Check sheet for the modelled part. Datum: model origin and axes. Units: mm. A direction names the side the tool comes from. Coordinates: 2 decimals unless noted, no trailing zeros. Order: outer loops, then holes, each group sorted by start corner. A loop starts at its lowest first (then second) coordinate and runs counter-clockwise, first axis right, second up.
from build123d import *

# Parameters (mm, degrees)
BOSS_EXTRUDE1_DEPTH     = 2.999994
SKETCH3_R               = 3.375082345
SKETCH3_R_2             = 2.3700486
BOSS_EXTRUDE2_DEPTH     = 3.302
SKETCH4_R               = 2.3700486
SKETCH4_R_2             = 1.524
BOSS_EXTRUDE3_DEPTH     = 2.237994
SKETCH5_R               = 3.556
SKETCH5_R_2             = 1.524049463
BOSS_EXTRUDE4_DEPTH     = 1.016
SKETCH6_R               = 1.524049463
CUT_EXTRUDE2_DEPTH      = 20.69939547
CUT_EXTRUDE3_START      = -4.015994
CUT_EXTRUDE3_OUTLINE_R  = 0.621776252
CUT_EXTRUDE3_DEPTH      = 4.015994
CUT_EXTRUDE4_DEPTH      = 21.047545727
CUT_EXTRUDE4_DEPTH_BACK = 3.302
SKETCH9_R               = 3.375082345
SKETCH10_R              = 2.54
CUT_EXTRUDE5_DEPTH      = 20.091339956


# Read off the part's stored shape, not the designer's step: Cut-Extrude3
with BuildPart() as part:
    # Sketch1 → Boss-Extrude1 (new body)
    with BuildSketch(Plane(origin=(0, 0, 0), x_dir=(1, 0, 0), z_dir=(0, 1, 0))):
        with BuildLine():
            Line((-14.960824333, 6.251943389), (-1.121532733, 7.748689189))
            ThreePointArc((-1.121532733, 7.748689189), (-0.719755533, 7.770352511), (-0.317978333, 7.748689189))
            Line((-0.317978333, 7.748689189), (13.521313267, 6.251943389))
            ThreePointArc((13.521313267, 6.251943389), (15.530246603, 4.014889189), (13.521313267, 1.777834989))
            Line((13.521313267, 1.777834989), (-0.317978333, 0.281089189))
            ThreePointArc((-0.317978333, 0.281089189), (-0.719755533, 0.259425867), (-1.121532733, 0.281089189))
            Line((-1.121532733, 0.281089189), (-14.960824333, 1.777834989))
            ThreePointArc((-14.960824333, 1.777834989), (-16.96975767, 4.014889189), (-14.960824333, 6.251943389))
        make_face()
    extrude(amount=BOSS_EXTRUDE1_DEPTH)

    # Sketch3 → Boss-Extrude2 (add)
    with BuildSketch(Plane(origin=(0, 2.999994, 0), x_dir=(1, 0, 0), z_dir=(0, 1, 0))):
        with Locations(Location((-0.719755307, 4.013536412, 0), (0, 0, 90))):
            Circle(SKETCH3_R)
        with Locations(Location((-0.719755307, 4.013536412, 0), (0, 0, 90))):
            Circle(SKETCH3_R_2, mode=Mode.SUBTRACT)
    extrude(amount=BOSS_EXTRUDE2_DEPTH)

    # Sketch4 → Boss-Extrude3 (add)
    with BuildSketch(Plane.XZ):
        with Locations(Location((-0.719755307, -4.013536412, 0), (0, 0, 270))):
            Circle(SKETCH4_R)
        with Locations((-0.719755307, -4.013536412)):
            Circle(SKETCH4_R_2, mode=Mode.SUBTRACT)
    extrude(amount=-BOSS_EXTRUDE3_DEPTH)

    # Sketch5 → Boss-Extrude4 (add)
    with BuildSketch(Plane.XZ):
        with Locations(Location((-0.7197993, -4.014912249, 0), (0, 0, 270))):
            Circle(SKETCH5_R)
        with Locations(Location((-0.7197993, -4.014912249, 0), (0, 0, 270))):
            Circle(SKETCH5_R_2, mode=Mode.SUBTRACT)
    extrude(amount=BOSS_EXTRUDE4_DEPTH)

    # Sketch6 → Cut-Extrude2 (cut, through all)
    with BuildSketch(Plane.XZ):
        with Locations(Location((-0.7197993, -4.014912249, 0), (0, 0, 270))):
            Circle(SKETCH6_R)
    extrude(amount=-CUT_EXTRUDE2_DEPTH, mode=Mode.SUBTRACT)

    # Cut-Extrude3 outline → Cut-Extrude3 (cut)
    with BuildSketch(Plane(origin=(0, 2.999994, 0), x_dir=(1, 0, 0), z_dir=(0, 1, 0)).offset(CUT_EXTRUDE3_START)):
        with BuildLine():
            ThreePointArc((-4.086322125, 3.773935294), (-4.094643941, 3.977376451), (-4.090683041, 4.18094921))
            ThreePointArc((-4.090683041, 4.18094921), (-5.297734637, 3.964486038), (-4.086322125, 3.773935294))
        make_face()
        with BuildLine():
            ThreePointArc((2.654580903, 4.084501036), (2.655136179, 3.977643639), (2.652308378, 3.870822222))
            ThreePointArc((2.652308378, 3.870822222), (3.887678446, 3.964535259), (2.654580903, 4.084501036))
        make_face()
        with Locations((-6.664608508, 3.970614789)):
            Circle(CUT_EXTRUDE3_OUTLINE_R)
        with Locations((9.231780819, 3.970614789)):
            Circle(CUT_EXTRUDE3_OUTLINE_R)
        with Locations((11.220395333, 3.970614789)):
            Circle(CUT_EXTRUDE3_OUTLINE_R)
        with Locations((13.209009847, 3.970614789)):
            Circle(CUT_EXTRUDE3_OUTLINE_R)
        with Locations((7.243166305, 3.970614789)):
            Circle(CUT_EXTRUDE3_OUTLINE_R)
        with Locations((5.254551791, 3.970614789)):
            Circle(CUT_EXTRUDE3_OUTLINE_R)
        with Locations((-14.619066564, 3.970614789)):
            Circle(CUT_EXTRUDE3_OUTLINE_R)
        with Locations((-12.63045205, 3.970614789)):
            Circle(CUT_EXTRUDE3_OUTLINE_R)
        with Locations((-10.641837536, 3.970614789)):
            Circle(CUT_EXTRUDE3_OUTLINE_R)
        with Locations((-8.653223022, 3.970614789)):
            Circle(CUT_EXTRUDE3_OUTLINE_R)
    extrude(amount=CUT_EXTRUDE3_DEPTH, mode=Mode.SUBTRACT)

    # Sketch9 → Cut-Extrude4 (cut, two sides: drawn at the far end of the back side and taken through both)
    with BuildSketch(Plane(origin=(0, 6.301994, 0), x_dir=(1, 0, 0), z_dir=(0, 1, 0)).offset(-CUT_EXTRUDE4_DEPTH_BACK)):
        with Locations((-0.719755307, 4.013536412)):
            Circle(SKETCH9_R)
    extrude(amount=CUT_EXTRUDE4_DEPTH + CUT_EXTRUDE4_DEPTH_BACK, mode=Mode.SUBTRACT)

    # Sketch10 → Cut-Extrude5 (cut, through all)
    with BuildSketch(Plane(origin=(0, 2.999994, 0), x_dir=(1, 0, 0), z_dir=(0, 1, 0))):
        with Locations(Location((-0.7197993, 4.014912249, 0), (0, 0, 270))):
            Circle(SKETCH10_R)
    extrude(amount=-CUT_EXTRUDE5_DEPTH, mode=Mode.SUBTRACT)


solid = part.part
(1) Cross-section at D-D (y = -0.3). Enter the section's corners in (x, z), and give its area (3 significant figures).
Filled in:
outline: (-4.25, -4.43) arc R3.56 ccw to (2.82, -4.4) arc R0.62 cw to (2.65, -4.08) arc R3.38 ccw to (2.65, -3.87) arc R0.62 cw to (2.81, -3.55) arc R3.56 ccw to (-4.24, -3.53) arc R0.62 cw to (-4.09, -3.77) arc R3.38 ccw to (-4.09, -4.18) arc R0.62 cw to start; hole circle Ø5.08 at (-0.72, -4.01)
area: 19.2 mm2
(2) Tool access check on faces 1 (the cylindrical face through (-0.78, -0.5, -7.57)), 2 (the cylindrical face through (-0.63, -0.5, -0.46)), 3 (the cylindrical face through (15.53, 1.48, -4.06)). Record the directions out of +Z, -Z, +X, -X, +Y, -Y that give a thin tool (end or side, any length) a straight path to the whole face; none if there is none.
Filled in:
face 1: -Z, -Y
face 2: +Z, -Y
face 3: +X, +Y, -Y
(3) Cross-section at B-B (x = -9). Enter the section's corners in (y, z), and give its area (3 significant figures).
Filled in:
outline: (0, -6.9) - (3, -6.9) - (3, -4.49) - (0, -4.49) - close; (0, -3.45) - (3, -3.45) - (3, -1.13) - (0, -1.13) - close
area: 14.2 mm2
(4) Go/stop test with flat-tipped pins: P1, Ø1, axis at x = -2, z = -2.5, coming from the +Y side; P2, Ø1, axis at y = 0.5, z = -6, coming from the -X side; P3, Ø1.4, axis at x = -8.65, z = -3.97, coming from the -Y side; P4, Ø2, axis at y = 2, z = -2, coming from the -X side. Record where each tip stops, or that it passes through.
Filled in:
P1: passes through
P2: stops at x = -16.41
P3: stops at y = 0
P4: stops at x = -16.73
(5) Cross-section at A-A (z = -5.75). Enter the section's corners in (x, y), and give its area (3 significant figures).
Filled in:
outline: (-16.15, 0) - (-3.82, 0) - (-3.82, -1.02) - (-2.57, -1.02) - (-2.57, 3) - (-16.15, 3) - close; (1.14, -1.02) - (2.38, -1.02) - (2.38, 0) - (14.71, 0) - (14.71, 3) - (1.14, 3) - close
area: 84.0 mm2
(6) Release check for a two-part mould opening along Z. For faces 4 (the cylindrical face through (-16.97, 1.48, -3.97)), 5 (the cylindrical face through (-5.298, 1.41, -3.989)), 6 (the flat face through (6.5, 1.48, -7.01)) record: +Z half, -Z half, draft (parallel to the pull), parting line (faces both ways), or undercut.
Filled in:
face 4: parting line
face 5: undercut
face 6: -Z half
(7) Thickness scan on probe 1 along Y at (x, z) = (-12, -3.5); probe 2 along Z at (x, y) = (3, 0.05); probe 3 along X at (y, z) = (-0.55, -5.5). Record the ranges inside material, lowest first.
Filled in:
probe 1: y = 0 to 3
probe 2: z = -7.39 to -4.53, -3.41 to -0.64
probe 3: x = -3.95 to -2.78, 1.34 to 2.51
(8) Cross-section at C-C (y = 2.2). Count the separate pieces of the cut face and the enclosed holes in it, and give its area (3 significant figures).
Filled in:
separate pieces: 1
enclosed holes: 13
area: 150 mm2
